Verification items for the finished model (mm, model axes). Face numbers are marked on the shaded views. A direction names the side the tool comes from. Give positions to 0.01 mm unless a question says otherwise; leave off trailing zeros. Write each loop counter-clockwise with the first axis right and the second up, starting at its lowest first coordinate (ties: lowest second). Pieces come first, ordered by that corner, then holes. Notation, with made-up numbers: (45.25, -11) - (61.25, -11) arc R15 cw to (61.25, 3) - close; hole circle Ø8 at (27, -21.75). An arc over 180 degrees is marked (long way). Put each result on its own line as item: value.
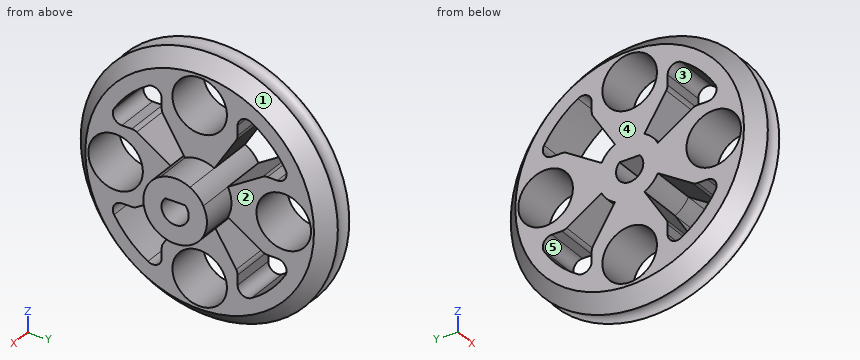
from build123d import *
from build123d import SkipClean  # not in build123d's __all__

# Parameters (mm, degrees)
F3_DEPTH = 25
F5_DEPTH = 25
F6_R     = 1
F7_R     = 3
F8_DEPTH = 25


with BuildPart() as f1:
    # F0 (on Top) → F1 (revolve)
    with BuildSketch(Plane.XY):
        with BuildLine():
            Line((-2.5, 12.5748384835), (-2.5, 0))
            Line((-2.5, 0), (6.5, 0))
            Line((6.5, 0), (6.5, 3.5))
            Line((6.5, 3.5), (2.5, 3.5))
            Line((2.5, 3.5), (2.5, 12.5748384835))
            Line((2.5, 12.5748384835), (0.9334766536, 14.1413618298))
            ThreePointArc((0.9334766536, 14.1413618298), (0, 13.5), (-0.9334766536, 14.1413618298))
            Line((-0.9334766536, 14.1413618298), (-2.5, 12.5748384835))
        make_face()
    revolve(axis=Axis((2, 0, 0), (1, 0, 0)))

    # F2 (on face) → F3 (cut)
    with BuildSketch(Plane(origin=(-2.5, 0, 0), x_dir=(0, -1, 0), z_dir=(-1, 0, 0))):
        with BuildLine():
            Line((-4.1763500472, 7.1763500472), (-4.1763500472, 10.1763500472))
            ThreePointArc((-4.1763500472, 10.1763500472), (-7.7781745931, 7.7781745931), (-10.1763500472, 4.1763500472))
            Line((-10.1763500472, 4.1763500472), (-7.1763500472, 4.1763500472))
            Line((-7.1763500472, 4.1763500472), (-3.1025807736, 1.6198742369))
            ThreePointArc((-3.1025807736, 1.6198742369), (-2.4748737342, 2.4748737342), (-1.6198742369, 3.1025807736))
            Line((-1.6198742369, 3.1025807736), (-4.1763500472, 7.1763500472))
        make_face()
        with BuildLine():
            ThreePointArc((10.1763500472, 4.1763500472), (7.7781745931, 7.7781745931), (4.1763500472, 10.1763500472))
            Line((4.1763500472, 10.1763500472), (4.1763500472, 7.1763500472))
            Line((4.1763500472, 7.1763500472), (1.6198742369, 3.1025807736))
            ThreePointArc((1.6198742369, 3.1025807736), (2.4748737342, 2.4748737342), (3.1025807736, 1.6198742369))
            Line((3.1025807736, 1.6198742369), (7.1763500472, 4.1763500472))
            Line((7.1763500472, 4.1763500472), (10.1763500472, 4.1763500472))
        make_face()
        with BuildLine():
            Line((-7.1763500472, -4.1763500472), (-10.1763500472, -4.1763500472))
            ThreePointArc((-10.1763500472, -4.1763500472), (-7.7781745931, -7.7781745931), (-4.1763500472, -10.1763500472))
            Line((-4.1763500472, -10.1763500472), (-4.1763500472, -7.1763500472))
            Line((-4.1763500472, -7.1763500472), (-1.6198742369, -3.1025807736))
            ThreePointArc((-1.6198742369, -3.1025807736), (-2.4748737342, -2.4748737342), (-3.1025807736, -1.6198742369))
            Line((-3.1025807736, -1.6198742369), (-7.1763500472, -4.1763500472))
        make_face()
        with BuildLine():
            Line((10.1763500472, -4.1763500472), (7.1763500472, -4.1763500472))
            Line((7.1763500472, -4.1763500472), (3.1025807736, -1.6198742369))
            ThreePointArc((3.1025807736, -1.6198742369), (2.4748737342, -2.4748737342), (1.6198742369, -3.1025807736))
            Line((1.6198742369, -3.1025807736), (4.1763500472, -7.1763500472))
            Line((4.1763500472, -7.1763500472), (4.1763500472, -10.1763500472))
            ThreePointArc((4.1763500472, -10.1763500472), (7.7781745931, -7.7781745931), (10.1763500472, -4.1763500472))
        make_face()
    with SkipClean():  # cleaning this boolean's faces spoils the solid; the shape is the same uncleaned
        extrude(amount=-F3_DEPTH, mode=Mode.SUBTRACT)

    # F4 (on face) → F5 (cut)
    with BuildSketch(Plane.YZ.offset(6.5)):
        with BuildLine():
            Line((1.1180339887, 1), (-1.1180339887, 1))
            ThreePointArc((-1.1180339887, 1), (0, -1.5), (1.1180339887, 1))
        make_face()
    with SkipClean():  # cleaning this boolean's faces spoils the solid; the shape is the same uncleaned
        extrude(amount=-F5_DEPTH, mode=Mode.SUBTRACT)

    # F6
    f6_edges = [f1.edges().sort_by_distance(p)[0] for p in [
        (0, -10.17635, 4.17635),
        (0, 4.17635, -10.17635),
        (0, -4.17635, -10.17635),
        (0, -10.17635, -4.17635),
        (0, 10.17635, -4.17635),
        (0, 10.17635, 4.17635),
        (0, 4.17635, 10.17635),
        (0, -4.17635, 10.17635),
        (0, -4.17635, -7.17635),
        (0, -7.17635, -4.17635),
        (0, 7.17635, -4.17635),
        (0, 4.17635, -7.17635),
        (0, -7.17635, 4.17635),
        (0, -4.17635, 7.17635),
        (0, 7.17635, 4.17635),
        (0, 4.17635, 7.17635),
    ]]
    fillet(f6_edges, radius=F6_R)

    # F7 (on face) → F8 (cut)
    with BuildSketch(Plane.YZ.offset(2.5)):
        with Locations((0, 9.25)):
            Circle(F7_R)
        with Locations((-9.25, 0)):
            Circle(F7_R)
        with Locations((9.25, 0)):
            Circle(F7_R)
        with Locations((0, -9.25)):
            Circle(F7_R)
    with SkipClean():  # cleaning this boolean's faces spoils the solid; the shape is the same uncleaned
        extrude(amount=-F8_DEPTH, mode=Mode.SUBTRACT)


solid = f1.part
Q1. Go/stop test with flat-tipped pins: pin 1 Ø2 at (x, z) = (5, 1) entering from +Y; pin 2 Ø6 at (y, z) = (-11, -6) entering from +X; pin 3 Ø2.5 at (x, y) = (3, 0) entering from -Z. Record where each tip stops, or that it passes through.
Answers follow:
pin 1: stops at y = 3.5
pin 2: stops at x = 2.5
pin 3: stops at z = -13.32
Q2. Scan lines: line 1 along Y through (x, z) = (0.5, -6.5); line 2 along Z through (x, y) = (0.4, 9.25); line 3 along Y through (x, z) = (0, -8). Record each from-to range of solid material in increasing order.
Answers follow:
line 1: y = -11.98 to -8.87, -3.75 to -1.2, 1.2 to 3.75, 8.87 to 11.98
line 2: z = -9.95 to -5.95, -4.46 to -3, 3 to 4.46, 5.95 to 9.95
line 3: y = -10.87 to -7.55, -4.18 to -2.73, 2.73 to 4.18, 7.55 to 10.87
Q3. Section check C-C, the plane x = 4.5. Record the cut outline in (y, z).
Answers follow:
outline: circle Ø7 at (0, 0); hole (-1.12, 1) arc R1.5 ccw (long way) to (1.12, 1) - close
Q4. Section check B-B, the plane z = 0. Record the cut outline in (x, y).
Answers follow:
outline: (-2.5, -12.57) - (-0.93, -14.14) arc R1 cw to (0.93, -14.14) - (2.5, -12.57) - (2.5, -12.25) - (-2.5, -12.25) - close; (-2.5, -6.25) - (2.5, -6.25) - (2.5, -3.5) - (6.5, -3.5) - (6.5, -1.5) - (-2.5, -1.5) - close; (-2.5, 1.5) - (6.5, 1.5) - (6.5, 3.5) - (2.5, 3.5) - (2.5, 6.25) - (-2.5, 6.25) - close; (-2.5, 12.25) - (2.5, 12.25) - (2.5, 12.57) - (0.93, 14.14) arc R1 cw to (-0.93, 14.14) - (-2.5, 12.57) - close
Q5. Section check D-D, the plane y = 9. Give the number of separate pieces and of enclosed holes in the cut face, plus the area to 3 significant figures.
Answers follow:
separate pieces: 4
enclosed holes: 0
area: 49.9 mm2
Q6. Set-up check for the marked faces 4 and 5: record each of +Z, -Z, +X, -X, +Y, -Y from which the full face is reachable in a straight line by a thin tool's end or side.
Answers follow:
face 4: +Z, -Z, -X, +Y, -Y
face 5: +X, -X
Q7. Release check for a two-part mould opening along Y. For the marked faces 1, 2 and 3 record: released by +Y, released by -Y, zero draft, split by the parting line, or undercut.
Answers follow:
face 1: split by the parting line
face 2: zero draft
face 3: undercut
Q8. Section check A-A, the plane y = 0. Record the cut outline in (x, z).
Answers follow:
outline: (-2.5, -12.57) - (-0.93, -14.14) arc R1 cw to (0.93, -14.14) - (2.5, -12.57) - (2.5, -12.25) - (-2.5, -12.25) - close; (-2.5, -6.25) - (2.5, -6.25) - (2.5, -3.5) - (6.5, -3.5) - (6.5, -1.5) - (-2.5, -1.5) - close; (-2.5, 1) - (6.5, 1) - (6.5, 3.5) - (2.5, 3.5) - (2.5, 6.25) - (-2.5, 6.25) - close; (-2.5, 12.25) - (2.5, 12.25) - (2.5, 12.57) - (0.93, 14.14) arc R1 cw to (-0.93, 14.14) - (-2.5, 12.57) - close
